Source: CAD feature listing. Evaluate the final solid. Frame: model axes, mm. Coordinates: 2 decimals unless noted, no trailing zeros. Write each loop counter-clockwise with the first axis right and the second up, starting at its lowest first coordinate (ties: lowest second). Pieces come first, ordered by that corner, then holes. Notation, with made-up numbers: (-39.75, -7.5) - (4.25, -7.5) arc R32 cw to (4.25, 25.5) - close; hole circle Ø6 at (27.25, 64). An arc over 180 degrees is marked (long way). One line per question, with ' | ' between items.
from build123d import *

# Parameters (mm, degrees)
SKETCH1_R           = 1.5
BOSS_EXTRUDE1_DEPTH = 2
SKETCH2_W           = 5
SKETCH2_H           = 26.4
BOSS_EXTRUDE2_DEPTH = 1.17


with BuildPart() as part:
    # Sketch1 → Boss-Extrude1 (new body)
    with BuildSketch(Plane(origin=(0, 0, 0), x_dir=(1, 0, 0), z_dir=(0, 1, 0))):
        Polygon((-3, 0), (0, 0), (10, 0), (10, 26.4), (42, 26.4), (42, 0), (52, 0), (55, 0), (55, 33), (-3, 33), align=None)
        with Locations(Location((0, 3.15, 0), (0, 0, 270))):
            Circle(SKETCH1_R, mode=Mode.SUBTRACT)
        with BuildLine():
            ThreePointArc((53.5, 3.15), (53.060660172, 2.089339828), (52, 1.65))
            ThreePointArc((52, 1.65), (50.939339828, 4.210660172), (53.5, 3.15))
        make_face(mode=Mode.SUBTRACT)
        with Locations(Location((2.5, 29.5, 0), (0, 0, 270))):
            Circle(SKETCH1_R, mode=Mode.SUBTRACT)
        with Locations(Location((49.5, 29.5, 0), (0, 0, 270))):
            Circle(SKETCH1_R, mode=Mode.SUBTRACT)
    extrude(amount=BOSS_EXTRUDE1_DEPTH)

    # Sketch2 → Boss-Extrude2 (add)
    with BuildSketch(Plane(origin=(0, 2, 0), x_dir=(1, 0, 0), z_dir=(0, 1, 0))):
        with Locations((7.5, 13.2)):
            Rectangle(SKETCH2_W, SKETCH2_H)
        with Locations((44.5, 13.2)):
            Rectangle(SKETCH2_W, SKETCH2_H)
    extrude(amount=BOSS_EXTRUDE2_DEPTH)


solid = part.part
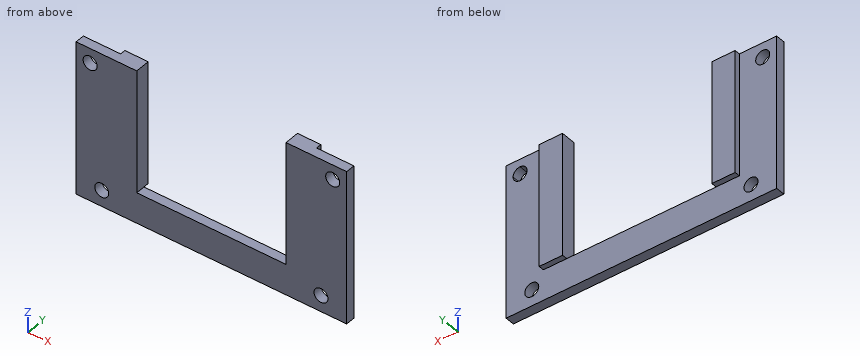
Item 1: Cut plane D-D on x = 18. Return loops of the section in (y, z).
Check sheet entries:
outline: (0, -33) - (2, -33) - (2, -26.4) - (0, -26.4) - close
Item 2: Cut plane A-A on x = 0. Return loops of the section in (y, z), and give its area (3 significant figures).
Check sheet entries:
outline: (0, -33) - (2, -33) - (2, -4.65) - (0, -4.65) - close; (0, -1.65) - (2, -1.65) - (2, 0) - (0, 0) - close | area: 60.0 mm²
Item 3: Cut plane C-C on z = -7. Return loops of the section in (x, y), and give its area (3 significant figures).
Check sheet entries:
outline: (-3, 0) - (10, 0) - (10, 3.17) - (5, 3.17) - (5, 2) - (-3, 2) - close; (42, 0) - (55, 0) - (55, 2) - (47, 2) - (47, 3.17) - (42, 3.17) - close | area: 63.7 mm²
Item 4: Pin query (flat end, axial travel): pin 1 Ø1.6 at (x, y) = (31.5, 0.5) entering from +Z; pin 2 Ø0.6 at (x, y) = (8, 2.5) entering from -Z; pin 3 Ø4 at (x, z) = (52, -3.15) entering from +Y. Return the tip coordinate at first contact, or that it passes through.
Check sheet entries:
pin 1: z = -26.4 | pin 2: z = -26.4 | pin 3: y = 2
Item 5: Ray query, line 1 along X through (y, z) = (1.4, -3.15); line 2 along X through (y, z) = (1.15, -29.5); line 3 along X through (y, z) = (2.35, -17). Return the intervals inside material, ascending. Write a range as [from, to].
Check sheet entries:
line 1: [-3, -1.5], [1.5, 10], [42, 50.5], [53.5, 55] | line 2: [-3, 1], [4, 48], [51, 55] | line 3: [5, 10], [42, 47]
Item 6: Cut plane B-B on y = 0.8. Return loops of the section in (x, z).
Check sheet entries:
outline: (-3, -33) - (55, -33) - (55, 0) - (42, 0) - (42, -26.4) - (10, -26.4) - (10, 0) - (-3, 0) - close; hole circle Ø3 at (0, -3.15); hole circle Ø3 at (2.5, -29.5); hole circle Ø3 at (49.5, -29.5); hole circle Ø3 at (52, -3.15)
